```python
from build123d import *

# Parameters (mm, degrees)
F0_R     = 4.25
F0_R_2   = 3.1
F1_DEPTH = 2
F2_DEPTH = 25


with BuildPart() as f1:
    # F0 (on Top) → F1 (new body)
    with BuildSketch(Plane.XY):
        Circle(F0_R)
        Circle(F0_R_2, mode=Mode.SUBTRACT)
    extrude(amount=F1_DEPTH)

    # F0 (on Top) → F2 (join)
    with BuildSketch(Plane.XY):
        Circle(F0_R_2)
        with BuildLine():
            Line((-1.35, 1.3), (1.35, 1.3))
            ThreePointArc((1.35, 1.3), (2.65, 0), (1.35, -1.3))
            Line((1.35, -1.3), (-1.35, -1.3))
            ThreePointArc((-1.35, -1.3), (-2.65, 0), (-1.35, 1.3))
        make_face(mode=Mode.SUBTRACT)
    extrude(amount=F2_DEPTH)


solid = f1.part
```
Part model, mm, in its own coordinate system. A direction names the side the tool comes from. Round coordinates to 2 decimals unless told otherwise and drop trailing zeros. Loops run counter-clockwise (first coordinate to the right, second up) from the corner with the lowest first, then second, coordinate; pieces in that order, holes last. Notation, with made-up numbers: (-7, 24.25) -> (1, 24.25) arc R19 cw to (1, 54.25) -> close; hole circle Ø5 at (12.25, 24.25). An arc over 180 degrees is marked (long way). Use CSV: the item, a comma, the result in double quotes. Start each with the question number.
1) Cut at D-D, the plane z = 1.75. Write the cut outline in (x, y), plus the area to 3 significant figures.
2) Cut at A-A, the plane y = 0. Write the cut outline in (x, z), plus the area to 3 significant figures.
3) Cut at C-C, the plane z = 11. Write the cut outline in (x, y), plus the area to 3 significant figures.
4) Drop flat-ended pins along their axis: P1, Ø1, axis at x = -1.5, z = 6, coming from the -Y side; P2, Ø5, axis at x = -0.5, z = 21.5, coming from the +Y side; P3, Ø1, axis at x = 1.5, y = -0.5, coming from the +Z side; P4, Ø1, axis at x = 0.5, z = 11.5, coming from the -Y side. Give the stop position or say it passes through.
5) Which spindle directions (+Z, -Z, +X, -X, +Y, -Y) get a long thin tool onto all of the face, cutting with end or side? Do faces 1 (the flat face through (0, -2, 0)), 2 (the cylindrical face through (2.65, 0.03, 12.32)), 3 (the cylindrical face through (1.43, -2.75, 13.34)). Say none if no direction does.
6) Wall check: L1, parallel to Y at x = 0, z = 20.75; L2, parallel to Z at x = 2.75, y = -1.5; L3, parallel to Y at x = 0.75, z = 16.5. Give the ranges that are in metal, low to high. Write a range as [from, to].
7) Cut at B-B, the plane x = 0. Write the cut outline in (y, z), plus the area to 3 significant figures.
Determined:
1,outline,"circle Ø8.5 at (0, 0); hole (-1.35, -1.3) -> (1.35, -1.3) arc R1.3 ccw to (1.35, 1.3) -> (-1.35, 1.3) arc R1.3 ccw to start"
1,area,"44.4 mm2"
2,outline,"(-4.25, 0) -> (-2.65, 0) -> (-2.65, 25) -> (-3.1, 25) -> (-3.1, 2) -> (-4.25, 2) -> close; (2.65, 0) -> (4.25, 0) -> (4.25, 2) -> (3.1, 2) -> (3.1, 25) -> (2.65, 25) -> close"
2,area,"27.1 mm2"
3,outline,"circle Ø6.2 at (0, 0); hole (-1.35, -1.3) -> (1.35, -1.3) arc R1.3 ccw to (1.35, 1.3) -> (-1.35, 1.3) arc R1.3 ccw to start"
3,area,"17.9 mm2"
4,P1,"stops at y = -2.93"
4,P2,"stops at y = 3.1"
4,P3,"passes through"
4,P4,"stops at y = -3.1"
5,face 1,"-Z, +X, -X, +Y, -Y"
5,face 2,"+Z, -Z"
5,face 3,"+Z"
6,L1,"y = [-3.1, -1.3], [1.3, 3.1]"
6,L2,"z = [0, 2]"
6,L3,"y = [-3.01, -1.3], [1.3, 3.01]"
7,outline,"(-4.25, 0) -> (-1.3, 0) -> (-1.3, 25) -> (-3.1, 25) -> (-3.1, 2) -> (-4.25, 2) -> close; (1.3, 0) -> (4.25, 0) -> (4.25, 2) -> (3.1, 2) -> (3.1, 25) -> (1.3, 25) -> close"
7,area,"94.6 mm2"
